Source: three-view drawing plus pictorial views. Frame: mm from the lowest corner of the part. Give positions to 0.01 mm unless a question says otherwise; leave off trailing zeros. Order: outer loops, then holes, each group sorted by start corner. A loop starts at its lowest first (then second) coordinate and runs counter-clockwise, first axis right, second up. Notation, with made-up numbers: (8, 0) -> (17, 0) arc R33 ccw to (17, 36) -> close; hole circle Ø6 at (-32, -3). An arc over 180 degrees is marked (long way). One line per question, with ' | ' between items.
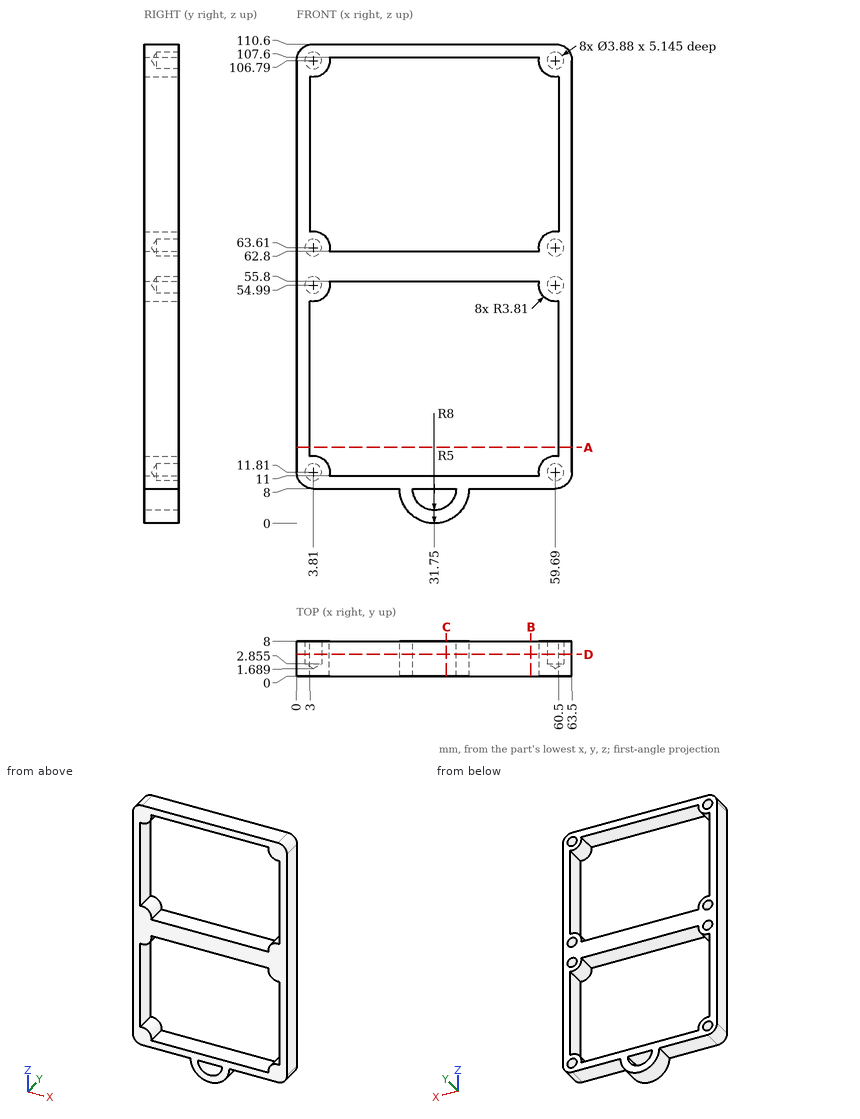
1) Contact query for a flat-ended pin moving along its axis: pin 1 Ø3.5 at (x, z) = (3.81, 11.81) entering from +Y. Output: stop coordinate, or through.
Check result:
pin 1: stops at y = 2.74
2) Section C-C on x = 34.5. Return loops of the section in (y, z).
Check result:
outline: (0, 0.49) -> (8, 0.49) -> (8, 3.82) -> (0, 3.82) -> close; (0, 8) -> (8, 8) -> (8, 11) -> (0, 11) -> close; (0, 55.8) -> (8, 55.8) -> (8, 62.8) -> (0, 62.8) -> close; (0, 107.6) -> (8, 107.6) -> (8, 110.6) -> (0, 110.6) -> close
3) Material intervals for probe 1 along Z at (x, y) = (32, 2); probe 2 along Z at (x, y) = (47.5, 5.5); probe 3 along X at (y, z) = (5.8, 63.61), sorted ascending. Write a range as from..to.
Check result:
probe 1: z = 0..3.01, 8..11, 55.8..62.8, 107.6..110.6 | probe 2: z = 8..11, 55.8..62.8, 107.6..110.6 | probe 3: x = 0..1.87, 5.75..7.62, 55.88..57.75, 61.63..63.5
4) Section B-B on x = 54. Return loops of the section in (y, z).
Check result:
outline: (0, 8) -> (8, 8) -> (8, 11) -> (0, 11) -> close; (0, 55.8) -> (8, 55.8) -> (8, 62.8) -> (0, 62.8) -> close; (0, 107.6) -> (8, 107.6) -> (8, 110.6) -> (0, 110.6) -> close
5) Section D-D on y = 5. Count the separate pieces of the cut face and the enclosed holes in it, plus the area to 3 significant figures.
Check result:
separate pieces: 1 | enclosed holes: 11 | area: 1,460 mm^2
6) Section A-A on z = 17.5. Return loops of the section in (x, y).
Check result:
outline: (0, 0) -> (3, 0) -> (3, 8) -> (0, 8) -> close; (60.5, 0) -> (63.5, 0) -> (63.5, 8) -> (60.5, 8) -> close
